The listing builds one solid part. Answer for the finished solid, in the listing's coordinates (mm). Give positions to 0.01 mm unless a question says otherwise; leave off trailing zeros. Write each loop counter-clockwise with the first axis right and the second up, starting at its lowest first coordinate (ties: lowest second). Pieces come first, ordered by that corner, then holes. Notation, with made-up numbers: (21.25, 49.5) - (75.25, 49.5) arc R19 ccw to (75.25, 59.5) - close; hole circle Ø3 at (28, 80.25). An arc over 180 degrees is marked (long way). Write each question's results on one line, items separated by ' | '. Start each with the question number.
Q1. Flat-ended cylindrical pins translate along their axes: pin 1 Ø3 at (x, y) = (0, 49.5) entering from +Z; pin 2 Ø5 at (x, y) = (-3, 52) entering from +Z; pin 3 Ø2 at (x, z) = (11.5, -11) entering from +Y. Find the tip coordinate at first contact, or state that the pin passes through.
Q2. Section B-B (z = 0) is taken. Determine the outline of the cut face in (x, y), plus the area to 3 significant figures.
Q3. Find the intervals of material crossed by probe 1 along X at (y, z) = (5.5, 18); probe 2 along X at (y, z) = (7, -17); probe 3 along Y at (x, z) = (0.5, 17), in increasing order.
Q4. For a pull along X with two mould halves and no side action, classify faces 1 (the face through (17.68, 21.89, -16.72)), 2 (the face through (-0.54, 55.7, 2.44)), 3 (the face through (0, 21, 21.59)) as pulls with the +X half, pulls with the -X half, needs draft (parallel to the pull), parting line crosses it, or undercut.
Q5. Section A-A (x = 0) is taken. Determine the outline of the cut face in (y, z), plus the area to 3 significant figures.
Q6. Section C-C (y = 62.5) is taken. Determine the outline of the cut face in (x, z), plus the area to 3 significant figures.
Q7. Section D-D (x = -5.5) is taken. Determine the outline of the cut face in (y, z), plus the area to 3 significant figures.
```python
from build123d import *

# Parameters (mm, degrees)
SKETCH1_W            = 43.18
SKETCH1_H            = 43.18
BOSS_EXTRUDE1_DEPTH  = 43.18
SKETCH2_R            = 2.5
BOSS_EXTRUDE2_DEPTH  = 25.4
SKETCH3_R            = 1.27
CUT_EXTRUDE1_DEPTH   = 43.18
LPATTERN1_COUNT      = 2
LPATTERN1_PITCH      = 35.9156
LPATTERN1_COUNT_DIR2 = 2
LPATTERN1_PITCH_DIR2 = 35.9156


with BuildPart() as part:
    # Sketch1 → Boss-Extrude1 (new body)
    with BuildSketch(Plane(origin=(0, 0, 0), x_dir=(1, 0, 0), z_dir=(0, 1, 0))):
        Rectangle(SKETCH1_W, SKETCH1_H)
    extrude(amount=BOSS_EXTRUDE1_DEPTH)

    # Sketch2 → Boss-Extrude2 (add)
    with BuildSketch(Plane(origin=(0, 43.18, 0), x_dir=(1, 0, 0), z_dir=(0, 1, 0))):
        Circle(SKETCH2_R)
    extrude(amount=BOSS_EXTRUDE2_DEPTH)

    # Sketch3 → Cut-Extrude1 (cut)
    with BuildSketch(Plane(origin=(0, 43.18, 0), x_dir=(1, 0, 0), z_dir=(0, 1, 0))):
        with Locations((-17.960512242, 17.960512242)):
            Circle(SKETCH3_R)
    cut_extrude1 = extrude(amount=-CUT_EXTRUDE1_DEPTH, mode=Mode.SUBTRACT)

    # LPattern1: Cut-Extrude1 2 × 2
    with Locations(*[(i * LPATTERN1_PITCH, 0, j * LPATTERN1_PITCH_DIR2) for i in range(LPATTERN1_COUNT) for j in range(LPATTERN1_COUNT_DIR2) if (i, j) != (0, 0)]):
        add(cut_extrude1, mode=Mode.SUBTRACT)


solid = part.part
```
Answers below:
1) pin 1: stops at z = 2.5 | pin 2: stops at z = 2.45 | pin 3: stops at y = 43.18
2) outline: (-21.59, 0) - (21.59, 0) - (21.59, 43.18) - (2.5, 43.18) - (2.5, 68.58) - (-2.5, 68.58) - (-2.5, 43.18) - (-21.59, 43.18) - close | area: 1,990 mm2
3) probe 1: x = -21.59 to -19.23, -16.69 to 16.69, 19.22 to 21.59 | probe 2: x = -21.59 to -18.79, -17.13 to 17.12, 18.79 to 21.59 | probe 3: y = 0 to 43.18
4) face 1: undercut | face 2: parting line crosses it | face 3: needs draft
5) outline: (0, -21.59) - (43.18, -21.59) - (43.18, -2.5) - (68.58, -2.5) - (68.58, 2.5) - (43.18, 2.5) - (43.18, 21.59) - (0, 21.59) - close | area: 1,990 mm2
6) outline: circle Ø5 at (0, 0) | area: 19.6 mm2
7) outline: (0, -21.59) - (43.18, -21.59) - (43.18, 21.59) - (0, 21.59) - close | area: 1,860 mm2
